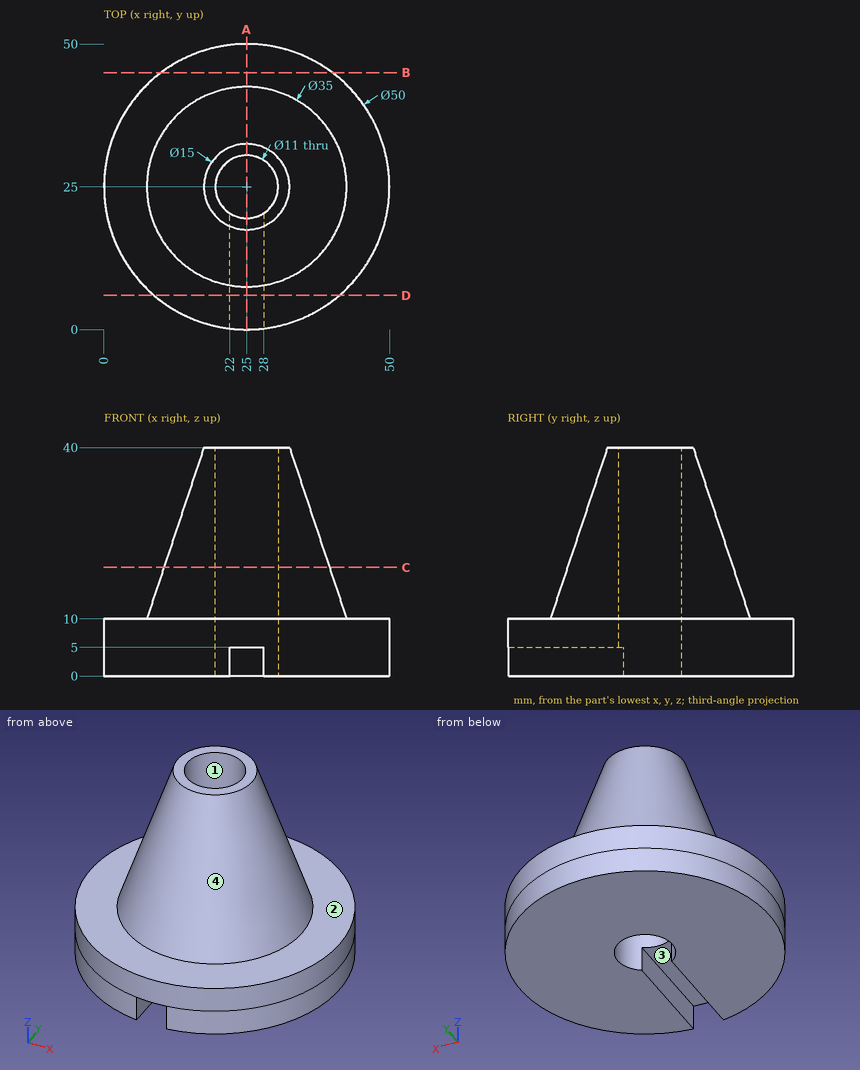
The figure shows three views and two pictorial views of one solid part (mm, origin at its lowest corner). Answer the questions. Give positions to 0.01 mm unless a question says otherwise; leave off trailing zeros. Loops run counter-clockwise (first coordinate to the right, second up) from the corner with the lowest first, then second, coordinate; pieces in that order, holes last. Notation, with made-up numbers: (88.25, 88) -> (143.25, 88) arc R10 ccw to (143.25, 95) -> close; hole circle Ø6 at (29.25, 48). An arc over 180 degrees is marked (long way). Use a Markdown table: item, result. Add a question column.
1. Section A-A on x = 25 is taken. Determine the outline of the cut face in (y, z), and give its area (4 significant figures).
2. Section C-C on z = 19 is taken. Determine the outline of the cut face in (x, y).
3. Determine the mould class of the marked faces 1, 2, 3 and 4 for opening direction X: released by +X, released by -X, zero draft, split by the parting line, or undercut.
4. Section B-B on y = 45 is taken. Determine the outline of the cut face in (x, z).
5. Section D-D on y = 6 is taken. Determine the outline of the cut face in (x, z), and give its area (3 significant figures).
6. Flat-ended cylindrical pins translate along their axes: pin 1 Ø1.5 at (y, z) = (14.5, 1.5) entering from -X; pin 2 Ø12 at (x, z) = (34, 34) entering from +Y; pin 3 Ø3 at (x, y) = (26, 14) entering from -Z. Find the tip coordinate at first contact, or state that the pin passes through.
7. Find the intervals of material crossed by probe 1 along Y at (x, z) = (25, 13); probe 2 along X at (y, z) = (25, 16); probe 3 along X at (y, z) = (25, 23.5), in increasing order.
Results below:
| question | item | result |
|---|---|---|
| 1 | outline | (0, 5) -> (19.5, 5) -> (19.5, 40) -> (17.5, 40) -> (7.5, 10) -> (0, 10) -> close; (30.5, 0) -> (50, 0) -> (50, 10) -> (42.5, 10) -> (32.5, 40) -> (30.5, 40) -> close |
| 1 | area | 712.5 mm^2 |
| 2 | outline | circle Ø29 at (25, 25); hole circle Ø11 at (25, 25) |
| 3 | face 1 | undercut |
| 3 | face 2 | zero draft |
| 3 | face 3 | undercut |
| 3 | face 4 | split by the parting line |
| 4 | outline | (10, 0) -> (40, 0) -> (40, 10) -> (10, 10) -> close |
| 5 | outline | (8.75, 0) -> (22, 0) -> (22, 5) -> (28, 5) -> (28, 0) -> (41.25, 0) -> (41.25, 10) -> (8.75, 10) -> close |
| 5 | area | 295 mm^2 |
| 6 | pin 1 | stops at x = 1.98 |
| 6 | pin 2 | stops at y = 34.85 |
| 6 | pin 3 | stops at z = 5 |
| 7 | probe 1 | y = 8.5 to 19.5, 30.5 to 41.5 |
| 7 | probe 2 | x = 9.5 to 19.5, 30.5 to 40.5 |
| 7 | probe 3 | x = 12 to 19.5, 30.5 to 38 |
